from build123d import *

# Parameters (mm, degrees)
F0_W     = 560
F0_H     = 130
F1_DEPTH = 21
F2_R     = 23
F2_W     = 42.5
F2_H     = 42.5
F3_DEPTH = 1


with BuildPart() as f1:
    # F0 (on Top) → F1 (new body)
    with BuildSketch(Plane.XY):
        with Locations((280, 65)):
            Rectangle(F0_W, F0_H)
    extrude(amount=F1_DEPTH)

    # F2 (on face) → F3 (cut)
    with BuildSketch(Plane.XY.offset(21)):
        with Locations((280, 65)):
            Circle(F2_R)
        with Locations((480, 65)):
            Rectangle(F2_W, F2_H)
    extrude(amount=-F3_DEPTH, mode=Mode.SUBTRACT)


solid = f1.part
Model file for the job. Use its own axes, mm. A direction names the side the tool comes from. Give positions to 0.01 mm unless a question says otherwise; leave off trailing zeros. Write each loop counter-clockwise with the first axis right and the second up, starting at its lowest first coordinate (ties: lowest second). Pieces come first, ordered by that corner, then holes. Notation, with made-up numbers: M 46.25,77.5 L 56.25,77.5 A17 cw 56.25,97.5 Z; hole C 71,87 d6. An arc over 180 degrees is marked long. One line per item, written item: value. Start each with the question number.
Q1. Probe probe 1 along Y at (x, z) = (280, 20.6). List the from-to ranges inside material, lowest first. Write a range as [from, to].
Q2. 3-axis set-ups, long thin cutter, end or side, ignore diameter. For faces 1 (the flat face through (280, 65, 20)), 2 (the flat face through (0, 64, 10)): which of +Z, -Z, +X, -X, +Y, -Y reach the whole face in a straight line?
Q3. Drop a flat-ended pin along its axis: pin 1 Ø14 at (x, y) = (284, 71.5) entering from +Z. Give the stop position or say it passes through.
Q4. Two-plate mould, pull along X, no slides. Class faces 3 (the flat face through (560, 64, 10)), 4 (the flat face through (276, 66, 0)), 5 (the flat face through (480, 65, 20)): +X half, -X half, draft (parallel to the pull), parting line (faces both ways), or undercut.
Q5. Saw through at B-B, the plane x = 280. Write the cut outline in (y, z).
Q6. Saw through at A-A, the plane x = 475. Write the cut outline in (y, z), plus the area to 3 significant figures.
Output values:
1. probe 1: y = [0, 42], [88, 130]
2. face 1: +Z
2. face 2: +Z, -Z, -X, +Y, -Y
3. pin 1: stops at z = 20
4. face 3: +X half
4. face 4: draft
4. face 5: undercut
5. outline: M 0,0 L 130,0 L 130,21 L 88,21 L 88,20 L 42,20 L 42,21 L 0,21 Z
6. outline: M 0,0 L 130,0 L 130,21 L 86.25,21 L 86.25,20 L 43.75,20 L 43.75,21 L 0,21 Z
6. area: 2,690 mm²
